For this review, use the dimensioned drawing (mm, ordinates from the lowest corner) and the shaded views. Round coordinates to 2 decimals unless told otherwise and drop trailing zeros. Order: outer loops, then holes, each group sorted by start corner. A loop starts at its lowest first (then second) coordinate and runs counter-clockwise, first axis right, second up. Notation, with made-up numbers: M -16,35.25 L 11,35.25 A18 cw 11,62.25 Z; hole C 29.25,-31 d6. An arc over 180 degrees is marked long. Use a Markdown table: item, result. Add a question column.
1. To check wall thickness, follow probe 1 along Y at (x, z) = (36, 15); probe 2 along Z at (x, y) = (63.5, 4.95); probe 3 along Z at (x, y) = (66, 2.5). State the ranges of each line that lie inside material, in increasing order.
2. Consider section B-B on z = 75. State the section outline as (x, y) points, then the cut area to 3 significant figures.
3. Consider section A-A on x = 60. State the section outline as (y, z) points, then the cut area to 3 significant figures.
4. Consider section C-C on y = 1.1. State the section outline as (x, z) points (3 decimals).
5. Insertion check: P1, Ø2, axis at y = 3, z = 93, coming from the +X side; P2, Ø12, axis at x = 107, z = 44, coming from the +Y side. Each pin has a flat end and moves straight along its axis. Give the tip position at first contact, or say it passes through.
6. Consider section D-D on x = 113.5. State the section outline as (y, z) points, then the cut area to 3 significant figures.
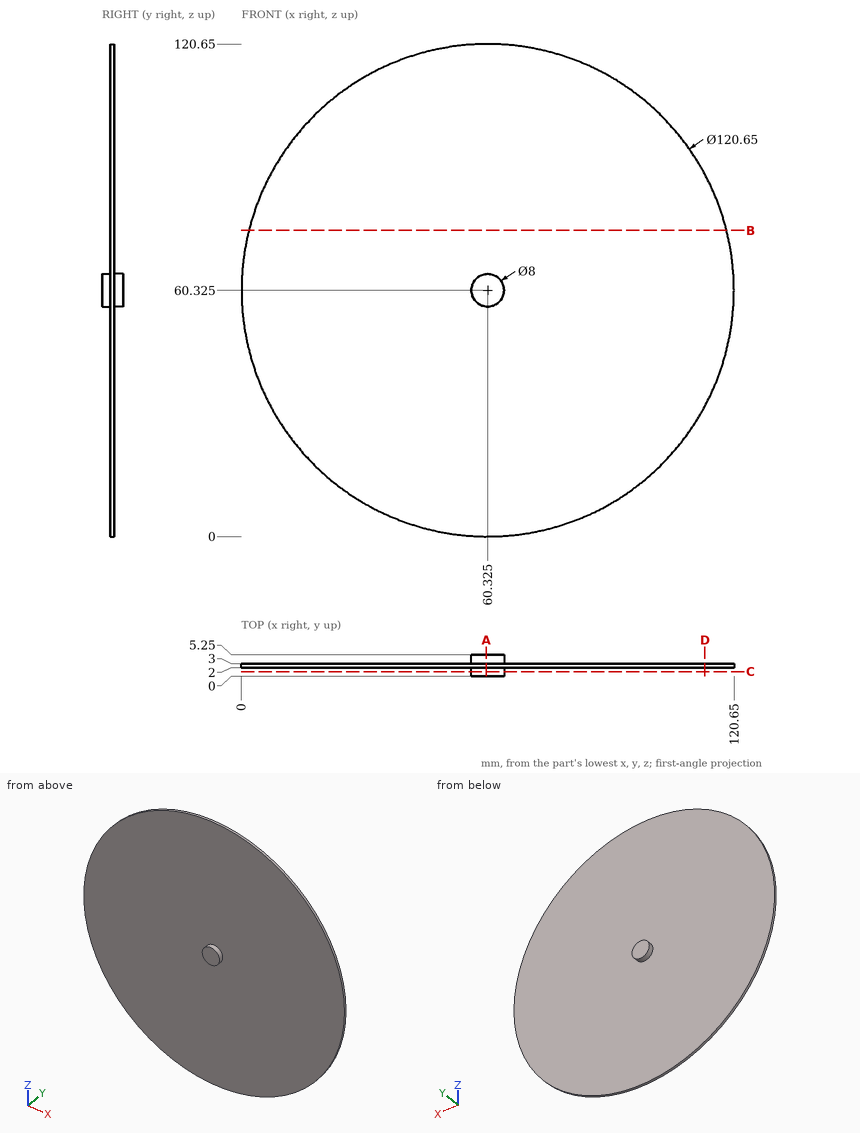
Answer block:
| question | item | result |
|---|---|---|
| 1 | probe 1 | 2 to 3 |
| 1 | probe 2 | 57.89 to 62.76 |
| 1 | probe 3 | 0.27 to 120.38 |
| 2 | outline | M 1.81,2 L 118.84,2 L 118.84,3 L 1.81,3 Z |
| 2 | area | 117 mm^2 |
| 3 | outline | M 0,56.34 L 2,56.34 L 2,0 L 3,0 L 3,56.34 L 5.25,56.34 L 5.25,64.31 L 3,64.31 L 3,120.65 L 2,120.65 L 2,64.31 L 0,64.31 Z |
| 3 | area | 155 mm^2 |
| 4 | outline | C 60.325,60.325 d8 |
| 5 | P1 | x = 111.67 |
| 5 | P2 | y = 3 |
| 6 | outline | M 2,31.84 L 3,31.84 L 3,88.81 L 2,88.81 Z |
| 6 | area | 57.0 mm^2 |
